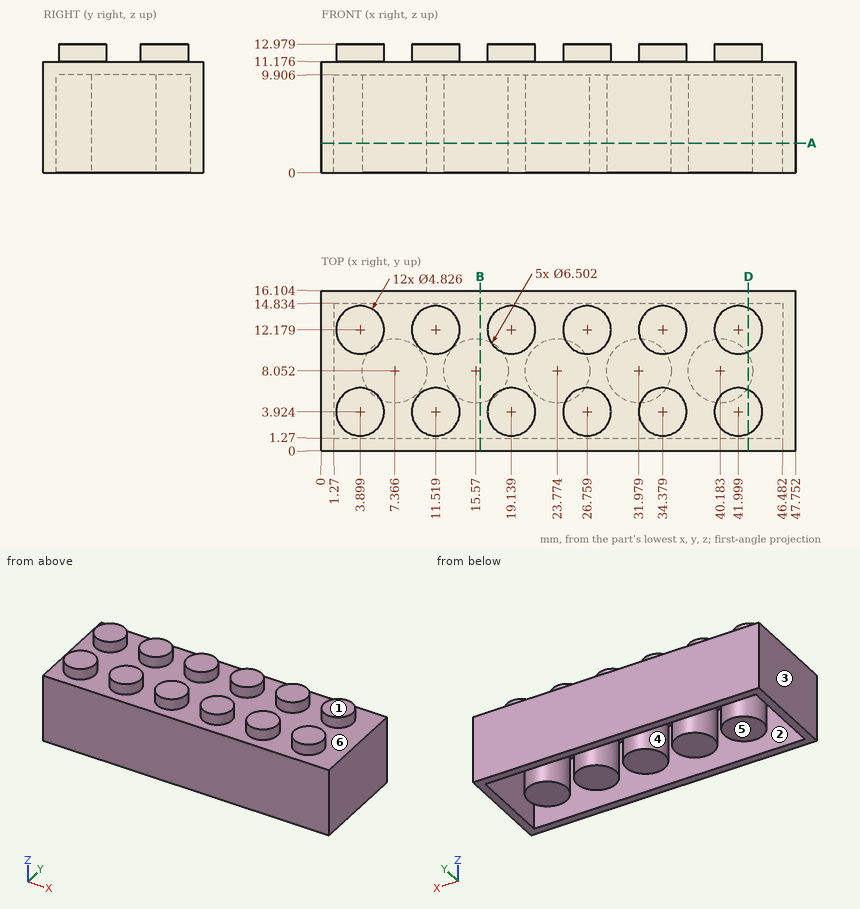
The figure shows three views and two pictorial views of one solid part (mm, origin at its lowest corner). Answer the questions. A direction names the side the tool comes from. Coordinates: 2 decimals unless noted, no trailing zeros. Loops run counter-clockwise (first coordinate to the right, second up) from the corner with the lowest first, then second, coordinate; pieces in that order, holes last. Notation, with made-up numbers: (-17, 42.5) - (7, 42.5) arc R30 cw to (7, 70.5) - close; hole circle Ø7 at (48.25, 36). An arc over 180 degrees is marked (long way). Answer in a Markdown table with one row per item.
Q1. Find section B-B on x = 16. Write down the section's boundary in (y, z) (1 decimal).
Here are the results:
| item | result |
|---|---|
| outline | (0, 0) - (1.3, 0) - (1.3, 9.9) - (4.8, 9.9) - (4.8, 0) - (11.3, 0) - (11.3, 9.9) - (14.8, 9.9) - (14.8, 0) - (16.1, 0) - (16.1, 11.2) - (0, 11.2) - close |
Q2. For the marked faces 4, 5 and 6, determine the directions among +Z, -Z, +X, -X, +Y, -Y from which every point of the face is accessible in a straight line to the end or side of a thin tool.
Here are the results:
| item | result |
|---|---|
| face 4 | -Z |
| face 5 | -Z, +X, -X, +Y, -Y |
| face 6 | +Z |
Q3. Find section D-D on x = 43. Write down the section's boundary in (y, z) (1 decimal).
Here are the results:
| item | result |
|---|---|
| outline | (0, 0) - (1.3, 0) - (1.3, 9.9) - (6.4, 9.9) - (6.4, 0) - (9.7, 0) - (9.7, 9.9) - (14.8, 9.9) - (14.8, 0) - (16.1, 0) - (16.1, 11.2) - (14.4, 11.2) - (14.4, 13) - (10, 13) - (10, 11.2) - (6.1, 11.2) - (6.1, 13) - (1.7, 13) - (1.7, 11.2) - (0, 11.2) - close |
Q4. Find section A-A on z = 3. Write down the section's boundary in (x, y) (1 decimal).
Here are the results:
| item | result |
|---|---|
| outline | (0, 0) - (47.8, 0) - (47.8, 16.1) - (0, 16.1) - close; circle Ø6.5 at (7.4, 8.1); circle Ø6.5 at (15.6, 8.1); circle Ø6.5 at (23.8, 8.1); circle Ø6.5 at (32, 8.1); circle Ø6.5 at (40.2, 8.1); hole (1.3, 1.3) - (46.5, 1.3) - (46.5, 14.8) - (1.3, 14.8) - close |
Q5. Straight lines are drawn through the part: line 1 along X through (y, z) = (2.75, 9); line 2 along Y through (x, z) = (41, 2.75) (1 decimal); line 3 along Y through (x, z) = (38, 3.25) (1 decimal). For each, find the intervals that lie inside material, in ascending order. Write a range as [from, to].
Here are the results:
| item | result |
|---|---|
| line 1 | x = [0, 1.27], [46.48, 47.75] |
| line 2 | y = [0, 1.3], [4.9, 11.2], [14.8, 16.1] |
| line 3 | y = [0, 1.3], [5.6, 10.5], [14.8, 16.1] |
Q6. The mould has two halves that part along X. Classify the marked faces 1, 2 and 3: pulls with the +X half, pulls with the -X half, needs draft (parallel to the pull), parting line crosses it, or undercut.
Here are the results:
| item | result |
|---|---|
| face 1 | needs draft |
| face 2 | undercut |
| face 3 | pulls with the -X half |
